Part model, mm, in its own coordinate system. A direction names the side the tool comes from. Coordinates: 2 decimals unless noted, no trailing zeros. Loops run counter-clockwise (first coordinate to the right, second up) from the corner with the lowest first, then second, coordinate; pieces in that order, holes last. Notation, with made-up numbers: (54.25, -7.75) - (112.25, -7.75) arc R21 cw to (112.25, 30.25) - close; hole circle Ø3 at (-21.75, -13). An arc over 180 degrees is marked (long way). Answer as CSV lines item,"result".
from build123d import *

# Parameters (mm, degrees)
SKETCH1_W           = 80
SKETCH1_H           = 60
SKETCH1_R           = 24.25
BOSS_EXTRUDE1_DEPTH = 20
BOSS_EXTRUDE3_DEPTH = 15
SKETCH5_R           = 2.1
CUT_EXTRUDE2_DEPTH  = 10
SKETCH6_W           = 80
SKETCH6_H           = 20
BOSS_EXTRUDE4_DEPTH = 2
BOSS_EXTRUDE6_DEPTH = 50
SKETCH9_R           = 2.1
CUT_EXTRUDE3_DEPTH  = 100.619275243
SKETCH12_W          = 80
SKETCH12_H          = 70
SKETCH12_R          = 1.65
BOSS_EXTRUDE8_DEPTH = 8
BOSS_EXTRUDE9_DEPTH = 15
CUT_EXTRUDE4_START  = -10
SKETCH14_R          = 2.1
CUT_EXTRUDE4_DEPTH  = 10
SKETCH16_R          = 2
CUT_EXTRUDE5_DEPTH  = 3
CIRPATTERN1_COUNT   = 3
FILLET1_R           = 3
CUT_EXTRUDE6_DEPTH  = 5


with BuildPart() as part:
    # Sketch1 → Boss-Extrude1 (new body)
    with BuildSketch(Plane.XY):
        Rectangle(SKETCH1_W, SKETCH1_H)
        Circle(SKETCH1_R, mode=Mode.SUBTRACT)
    extrude(amount=BOSS_EXTRUDE1_DEPTH)

    # Sketch4 → Boss-Extrude3 (add)
    with BuildSketch(Plane(origin=(40, 0, 0), x_dir=(0, 0, -1), z_dir=(1, 0, 0))):
        Polygon((-20, 30), (0, 30), (20, 30), (20, 20), (0, 20), (-20, 20), align=None)
    boss_extrude3 = extrude(amount=BOSS_EXTRUDE3_DEPTH)

    # Sketch5 → Cut-Extrude2 (cut)
    with BuildSketch(Plane(origin=(0, 30, 0), x_dir=(1, 0, 0), z_dir=(0, 1, 0))):
        with Locations(Location((47.5, -10, 0), (0, 0, 270))):
            Circle(SKETCH5_R)
        with Locations(Location((47.5, 10, 0), (0, 0, 270))):
            Circle(SKETCH5_R)
        Polygon((46, -20), (55, -15), (55, -20), align=None)
    cut_extrude2 = extrude(amount=-CUT_EXTRUDE2_DEPTH, mode=Mode.SUBTRACT)

    # Sketch6 → Boss-Extrude4 (add)
    with BuildSketch(Plane(origin=(0, -30, 0), x_dir=(-1, 0, 0), z_dir=(0, -1, 0))):
        with Locations((0, -10)):
            Rectangle(SKETCH6_W, SKETCH6_H)
    boss_extrude4 = extrude(amount=BOSS_EXTRUDE4_DEPTH)

    # Sketch8 → Boss-Extrude6 (add)
    with BuildSketch(Plane(origin=(0, 0, 0), x_dir=(-1, 0, 0), z_dir=(0, 0, -1))):
        Polygon((-40, -11), (-19, -32), (-40, -32), align=None)
    boss_extrude6 = extrude(amount=BOSS_EXTRUDE6_DEPTH)

    # Sketch9 → Cut-Extrude3 (cut, through all)
    with BuildSketch(Plane(origin=(40, 0, 0), x_dir=(0, 0, -1), z_dir=(1, 0, 0))):
        with Locations((27, -28)):
            Circle(SKETCH9_R)
    cut_extrude3 = extrude(amount=-CUT_EXTRUDE3_DEPTH, mode=Mode.SUBTRACT)

    # Sketch12 → Boss-Extrude8 (add)
    with BuildSketch(Plane.XZ.offset(32)):
        with Locations((0, -15)):
            Rectangle(SKETCH12_W, SKETCH12_H)
        with Locations(Location((-8, -8.3, 0), (0, 0, 270))):
            Circle(SKETCH12_R, mode=Mode.SUBTRACT)
        with Locations(Location((8, -8.3, 0), (0, 0, 270))):
            Circle(SKETCH12_R, mode=Mode.SUBTRACT)
        with Locations(Location((8, -38.3, 0), (0, 0, 270))):
            Circle(SKETCH12_R, mode=Mode.SUBTRACT)
        with Locations(Location((-8, -38.3, 0), (0, 0, 270))):
            Circle(SKETCH12_R, mode=Mode.SUBTRACT)
    extrude(amount=BOSS_EXTRUDE8_DEPTH)

    # Mirror1: Boss-Extrude3, Cut-Extrude2, Boss-Extrude4, Boss-Extrude6, Cut-Extrude3 across plane
    add(boss_extrude3.mirror(Plane(origin=(0, 0, 0), x_dir=(0, 0, 1), z_dir=(1, 0, 0))))
    add(cut_extrude2.mirror(Plane(origin=(0, 0, 0), x_dir=(0, 0, 1), z_dir=(1, 0, 0))), mode=Mode.SUBTRACT)
    add(boss_extrude4.mirror(Plane(origin=(0, 0, 0), x_dir=(0, 0, 1), z_dir=(1, 0, 0))))
    add(boss_extrude6.mirror(Plane(origin=(0, 0, 0), x_dir=(0, 0, 1), z_dir=(1, 0, 0))))
    add(cut_extrude3.mirror(Plane(origin=(0, 0, 0), x_dir=(0, 0, 1), z_dir=(1, 0, 0))), mode=Mode.SUBTRACT)

    # Sketch13 → Boss-Extrude9 (add)
    with BuildSketch(Plane.ZY.offset(40)):
        Polygon((20, -40), (0, -40), (-20, -40), (-20, -32), (0, -32), (20, -32), align=None)
    boss_extrude9 = extrude(amount=BOSS_EXTRUDE9_DEPTH)

    # Sketch14 → Cut-Extrude4 (cut)
    with BuildSketch(Plane.XZ.offset(40).offset(CUT_EXTRUDE4_START)):
        with Locations(Location((-47.5, 10, 0), (0, 0, 90))):
            Circle(SKETCH14_R)
        with Locations(Location((-47.5, -10, 0), (0, 0, 90))):
            Circle(SKETCH14_R)
    cut_extrude4 = extrude(amount=CUT_EXTRUDE4_DEPTH, mode=Mode.SUBTRACT)

    # Mirror2: Boss-Extrude9, Cut-Extrude4 across plane
    add(boss_extrude9.mirror(Plane(origin=(0, 0, 0), x_dir=(0, 0, 1), z_dir=(1, 0, 0))))
    add(cut_extrude4.mirror(Plane(origin=(0, 0, 0), x_dir=(0, 0, 1), z_dir=(1, 0, 0))), mode=Mode.SUBTRACT)

    # Sketch16 → Cut-Extrude5 (cut)
    with BuildSketch(Plane.XY.offset(20)):
        with Locations((0, -30)):
            Circle(SKETCH16_R)
    cut_extrude5 = extrude(amount=-CUT_EXTRUDE5_DEPTH, mode=Mode.SUBTRACT)

    # CirPattern1: Cut-Extrude5 ×3 about axis
    cirpattern1_axis = Axis((0, 0, 0), (0, 0, 1))
    for i in range(1, CIRPATTERN1_COUNT):
        add(cut_extrude5.rotate(cirpattern1_axis, i * 360 / CIRPATTERN1_COUNT), mode=Mode.SUBTRACT)

    # Fillet1
    fillet1_edges = [part.edges().sort_by_distance(p)[0] for p in [
        (-40, 20, 10),
        (-40, -32, 0),
        (-40, -36, -20),
        (40, 20, 10),
        (40, -32, 0),
        (40, -36, -20),
    ]]
    fillet(fillet1_edges, radius=FILLET1_R)

    # Sketch17 → Cut-Extrude6 (cut)
    with BuildSketch(Plane.XY.offset(17)):
        Polygon((-3.6, -32.078460969), (-3.6, -40), (3.6, -40), (3.6, -32.078460969), (3.6, -27.921539031), (0, -25.843078062), (-3.6, -27.921539031), align=None)
        Polygon((29.323026539, 17.47169345), (25.511345008, 19.130332624), (22.169080583, 16.658639174), (22.638497688, 12.52830655), (26.450179219, 10.869667376), (42.459549451, 3.903248909), (45.851836141, 11.698986963), align=None)
        Polygon((-21.915647081, 15.868815152), (-24.70062059, 18.954900464), (-28.765735623, 18.086085312), (-43.679312497, 14.998912364), (-42.219854604, 7.948533961), (-27.260903637, 11.045099536), (-23.195788604, 11.913914688), align=None)
    extrude(amount=-CUT_EXTRUDE6_DEPTH, mode=Mode.SUBTRACT)


solid = part.part
Q1. Saw through at B-B (y = 0). Give the cut face in (x, z), then the cut area to 3 significant figures.
Results:
outline,"(-40, 0) - (-24.25, 0) - (-24.25, 20) - (-40, 20) - close; (24.25, 0) - (40, 0) - (40, 20) - (24.25, 20) - close"
area,"630 mm^2"
Q2. Two-plate mould, pull along X, no slides. Class faces 1 (the face through (-55, -36, 0)), 2 (the face through (-3.6, -34, 15)), 3 (the face through (55, -36, 0)): released by +X, released by -X, zero draft, split by the parting line, or undercut.
Results:
face 1,"released by -X"
face 2,"undercut"
face 3,"released by +X"
Q3. Saw through at A-A (z = 10). Count the separate pieces of the cut face and the enclosed holes in it, then the cut area to 3 significant figures.
Results:
separate pieces,"5"
enclosed holes,"1"
area,"4,150 mm^2"
Q4. Wall check: L1, parallel to X at y = 27.75, z = 10; L2, parallel to X at y = -35.5, z = -38.3; L3, parallel to Z at x = 47, y = 24. Give the ranges that are in metal, low to high.
Results:
L1,"x = -55 to -49.6, -45.4 to 45.4, 49.6 to 55"
L2,"x = -40 to -9.65, -6.35 to 6.35, 9.65 to 40"
L3,"z = -20 to -12.04, -7.96 to 7.96, 12.04 to 19.44"
Q5. Saw through at C-C (z = -13.5). Give the cut face in (x, y), then the cut area to 3 significant figures.
Results:
outline,"(-55, -40) - (55, -40) - (55, -32) - (43, -32) arc R3 cw to (40, -29) - (40, -11) - (19, -32) - (-19, -32) - (-40, -11) - (-40, -29) arc R3 cw to (-43, -32) - (-55, -32) - close; (-55, 20) - (-40, 20) - (-40, 30) - (-55, 30) - close; (40, 20) - (55, 20) - (55, 30) - (40, 30) - close"
area,"1,620 mm^2"
Q6. Which spindle directions (+Z, -Z, +X, -X, +Y, -Y) get a long thin tool onto all of the face, cutting with end or side? Do faces 4 (the face through (-40, -18, -15)), 5 (the face through (34.74, 15.58, 14.54)), 6 (the face through (-25.257, 11.473, 14.535)), 7 (the face through (0, -32, 19)), 8 (the face through (47, 20, -4)). Say none if no direction does.
Results:
face 4,"-Z, -X"
face 5,"none"
face 6,"-X"
face 7,"+Z"
face 8,"-Z, +X"
Q7. Saw through at D-D (x = -8). Give the cut face in (y, z).
Results:
outline,"(-40, -50) - (-32, -50) - (-32, -39.95) - (-40, -39.95) - close; (-40, -36.65) - (-32, -36.65) - (-32, -9.95) - (-40, -9.95) - close; (-40, -6.65) - (-32, -6.65) - (-32, 0) - (-22.89, 0) - (-22.89, 20) - (-40, 20) - close; (22.89, 0) - (30, 0) - (30, 20) - (22.89, 20) - close"
Q8. Flat gauge pins, fed straight in: pin 1 (11.5 mm diameter, centred on x = -29, y = 16, fed in from -Z); pin 2 (6 mm diameter, centred on y = -14, z = -39.5, fed in from -X); pin 3 (1.5 mm diameter, centred on x = 34.5, z = -5.5, fed in from +Y). Where does each tip first touch, or does it go through?
Results:
pin 1,"stops at z = 0"
pin 2,"stops at x = -40"
pin 3,"stops at y = -15.75"
